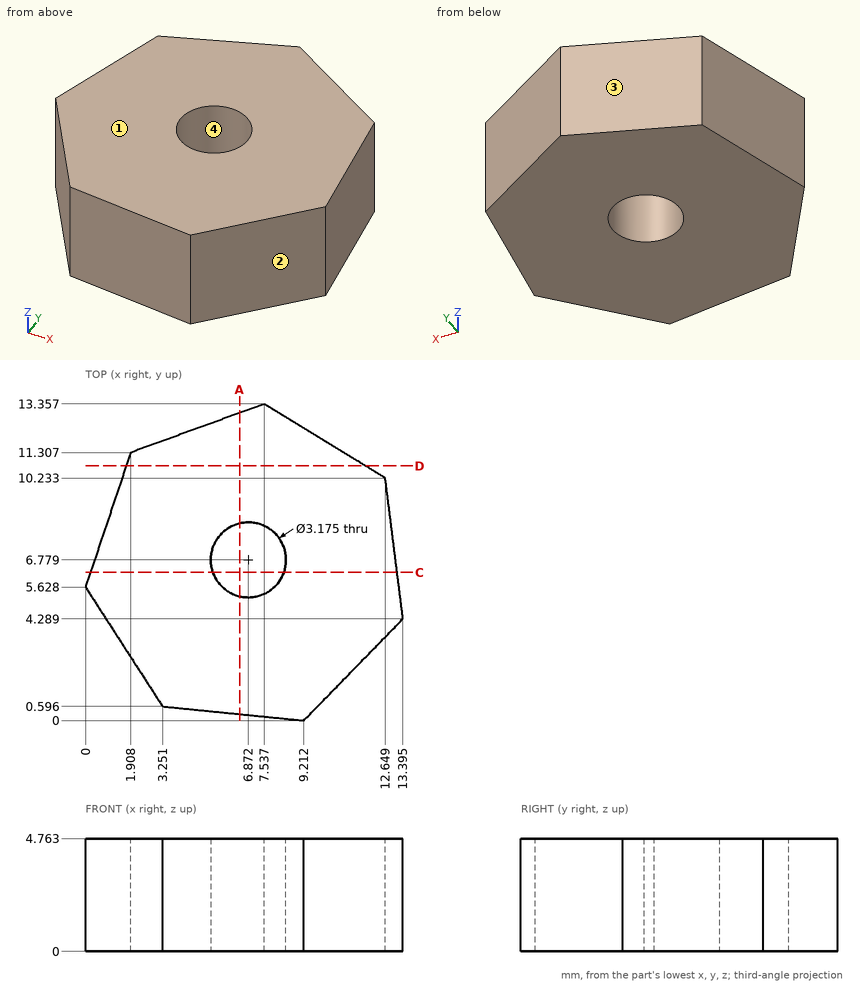
Part print with two shaded views. Sizes in mm from the minimum x, y, z corner. Coordinates: 2 decimals unless noted, no trailing zeros. Write each loop counter-clockwise with the first axis right and the second up, starting at its lowest first coordinate (ties: lowest second). Pieces come first, ordered by that corner, then holes. Notation, with made-up numbers: (34.5, -6.75) -> (83.5, -6.75) arc R14 cw to (83.5, 14.25) -> close; hole circle Ø6 at (65, 49.5). An arc over 180 degrees is marked (long way). Return JSON: item names as keys, results as strings. Group by question number.
Q1. Cut at D-D, the plane y = 10.75. Give the cut face in (x, z).
Q2. Cut at A-A, the plane x = 6.5. Give the cut face in (y, z) (1 decimal).
Q3. Pull direction Y, two halves, no side cores. Call the marked faces 1, 2, 3 and 4: released by +Y, released by -Y, zero draft, split by the parting line, or undercut.
Q4. Drill centre lines: line 1 (X direction, y = 5.75, z = 2.3) (1 decimal); line 2 (X direction, y = 7.75, z = 0.4) (1 decimal); line 3 (X direction, y = 5, z = 1.2) (1 decimal). Where is each one in solid material? Low to high.
Q5. Flat gauge pins, fed straight in: pin 1 (2 mm diameter, centred on y = 7, z = 2, fed in from +X); pin 2 (1.5 mm diameter, centred on y = 10.5, z = 4, fed in from +X); pin 3 (3 mm diameter, centred on x = 6.87, y = 6.78, fed in from +Z). Where does each tip first touch, or does it go through?
Q6. Cut at C-C, the plane y = 6.25. Give the cut face in (x, z) (1 decimal).
Returned:
{
 "1": {"outline": "(1.72, 0) -> (11.8, 0) -> (11.8, 4.76) -> (1.72, 4.76) -> close"},
 "2": {"outline": "(0.3, 0) -> (5.2, 0) -> (5.2, 4.8) -> (0.3, 4.8) -> close; (8.3, 0) -> (13, 0) -> (13, 4.8) -> (8.3, 4.8) -> close"},
 "3": {"face 1": "zero draft", "face 2": "released by -Y", "face 3": "released by +Y", "face 4": "undercut"},
 "4": {"line 1": "x = 0 to 5.7, 8.1 to 13.2", "line 2": "x = 0.7 to 5.6, 8.1 to 13", "line 3": "x = 0.4 to 13.3"},
 "5": {"pin 1": "stops at x = 13.18", "pin 2": "stops at x = 12.71", "pin 3": "passes through"},
 "6": {"outline": "(0.2, 0) -> (5.4, 0) -> (5.4, 4.8) -> (0.2, 4.8) -> close; (8.4, 0) -> (13.1, 0) -> (13.1, 4.8) -> (8.4, 4.8) -> close"}
}
